Answer from the drawing. Dimensions are ordinates in mm from the lowest x, y and z of the part. Coordinates: 2 decimals unless noted, no trailing zeros. Order: outer loops, then holes, each group sorted by start corner. A loop starts at its lowest first (then second) coordinate and runs counter-clockwise, first axis right, second up. Notation, with made-up numbers: (51.5, 38.5) -> (55.5, 38.5) arc R33 ccw to (55.5, 76.5) -> close; hole circle Ø3 at (52.5, 61). An arc over 180 degrees is marked (long way). Answer in a Markdown table with one row per item.
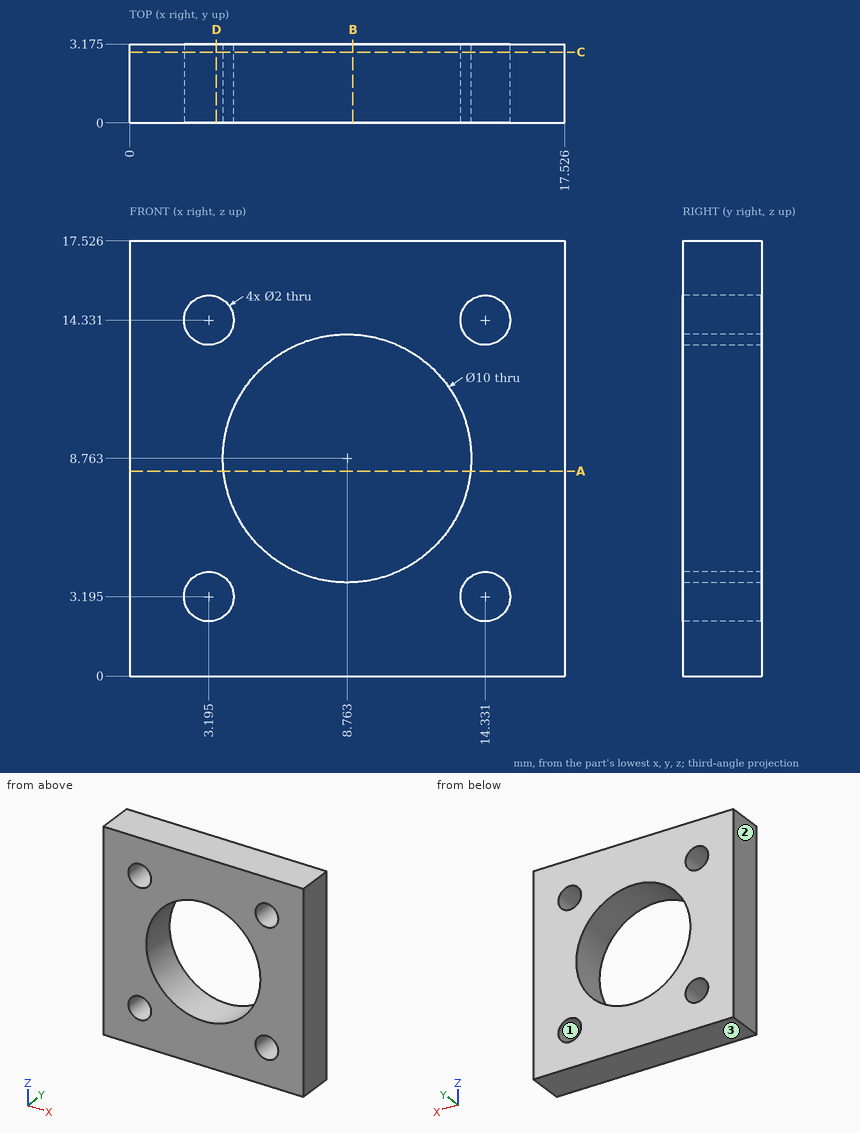
Q1. The part is cut by section B-B (x = 9). Write down the section's boundary in (y, z) (1 decimal), then the cut area to 3 significant figures.
Outcome:
| item | result |
|---|---|
| outline | (0, 0) -> (3.2, 0) -> (3.2, 3.8) -> (0, 3.8) -> close; (0, 13.8) -> (3.2, 13.8) -> (3.2, 17.5) -> (0, 17.5) -> close |
| area | 23.9 mm² |
Q2. Consider line 1 (X direction, y = 1.65, z = 14.25); line 2 (Z direction, x = 9, y = 1.7). Determine where each line is inside the solid, lowest interval first.
Outcome:
| item | result |
|---|---|
| line 1 | 0 to 2.2, 4.19 to 13.33, 15.33 to 17.53 |
| line 2 | 0 to 3.77, 13.76 to 17.53 |
Q3. The part is cut by section D-D (x = 3.5). Write down the section's boundary in (y, z) (1 decimal).
Outcome:
| item | result |
|---|---|
| outline | (0, 0) -> (3.2, 0) -> (3.2, 2.2) -> (0, 2.2) -> close; (0, 4.1) -> (3.2, 4.1) -> (3.2, 13.4) -> (0, 13.4) -> close; (0, 15.3) -> (3.2, 15.3) -> (3.2, 17.5) -> (0, 17.5) -> close |
Q4. The part is cut by section A-A (z = 8.25). Write down the section's boundary in (x, y) (1 decimal).
Outcome:
| item | result |
|---|---|
| outline | (0, 0) -> (3.8, 0) -> (3.8, 3.2) -> (0, 3.2) -> close; (13.7, 0) -> (17.5, 0) -> (17.5, 3.2) -> (13.7, 3.2) -> close |
Q5. The part is cut by section C-C (y = 2.85). Write down the section's boundary in (x, z) (1 decimal).
Outcome:
| item | result |
|---|---|
| outline | (0, 0) -> (17.5, 0) -> (17.5, 17.5) -> (0, 17.5) -> close; hole circle Ø2 at (3.2, 3.2); hole circle Ø2 at (3.2, 14.3); hole circle Ø10 at (8.8, 8.8); hole circle Ø2 at (14.3, 3.2); hole circle Ø2 at (14.3, 14.3) |
Q6. For a pull along Z with two mould halves and no side action, classify the marked faces 1, 2 and 3 as pulls with the +Z half, pulls with the -Z half, needs draft (parallel to the pull), parting line crosses it, or undercut.
Outcome:
| item | result |
|---|---|
| face 1 | undercut |
| face 2 | needs draft |
| face 3 | pulls with the -Z half |
